from build123d import *

# Parameters (mm, degrees)
BOSS_EXTRUDE1_DEPTH = 1.5


with BuildPart() as part:
    # Sketch1 → Revolve1 (revolve)
    with BuildSketch(Plane.XY, mode=Mode.PRIVATE) as revolve1_sk:
        with BuildLine():
            Line((0, 0), (1.775, 0))
            Line((1.775, 0), (1.775, 6.5))
            Line((1.775, 6.5), (2.775, 6.5))
            ThreePointArc((2.775, 6.5), (2.302554278, 6.609277193), (1.818611947, 6.640038943))
            Line((1.818611947, 6.640038943), (0, 6.640038943))
            Line((0, 6.640038943), (0, 0))
        make_face()
    revolve(revolve1_sk.sketch.rotate(Axis((0, 0, 0), (0, 1, 0)), 90), axis=Axis((0, 0, 0), (0, 1, 0)))

    # Sketch2 → Boss-Extrude1 (add)
    with BuildSketch(Plane(origin=(0, 6.640038943, 0), x_dir=(1, 0, 0), z_dir=(0, 1, 0))):
        Polygon((1.349267315, 1.604637118), (-0.71502285, 1.97081833), (-2.064290165, 0.366181213), (-1.349267315, -1.604637118), (0.71502285, -1.97081833), (2.064290165, -0.366181213), align=None)
    extrude(amount=BOSS_EXTRUDE1_DEPTH)

    # Sketch3 → Cut-Revolve1 (revolve, cut)
    with BuildSketch(Plane.XY, mode=Mode.PRIVATE) as cut_revolve1_sk:
        Polygon((1.11158303, 8.796006759), (2.422382115, 7.573543033), (2.422382115, 8.796006759), align=None)
    revolve(cut_revolve1_sk.sketch.rotate(Axis((0, 0, 0), (0, 1, 0)), 90), axis=Axis((0, 0, 0), (0, 1, 0)), mode=Mode.SUBTRACT)


solid = part.part
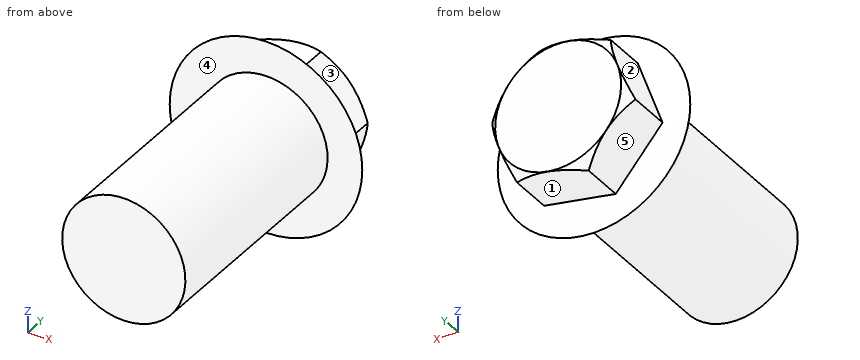
Geometry check sheet. Reference: the model listing, model coordinates, mm. Face numbers are marked on the shaded views. A direction names the side the tool comes from. Round coordinates to 2 decimals unless told otherwise and drop trailing zeros. Order: outer loops, then holes, each group sorted by start corner. A loop starts at its lowest first (then second) coordinate and runs counter-clockwise, first axis right, second up. Notation, with made-up numbers: M 73,85 L 124,85 A15 cw 124,112 Z; hole C 81.5,26.25 d4. An arc over 180 degrees is marked long. Write each question's results on one line, items separated by ' | '. Start each with the question number.
1. Material ranges on L1, parallel to Z at x = -0.6, y = 3.75; L2, parallel to X at y = 3.5, z = 0 (3 decimals); L3, parallel to X at y = 5.5, z = -0.35, recorded low to high. Write a range as from..to.
2. Set-up check for the marked faces 1, 2, 3, 4 and 5: record each of +Z, -Z, +X, -X, +Y, -Y from which the full face is reachable in a straight line by a thin tool's end or side.
3. Cross-section at A-A on y = 1.25. Record the boundary of the cut face in (x, z) (3 decimals), plus the area to 3 significant figures.
Resolved:
1) L1: -1.67..1.67 | L2: -1.775..1.775 | L3: -1.74..1.74
2) face 1: -Z, +X, +Y | face 2: +Z, -X, +Y | face 3: +Z, +X, +Y | face 4: -Y | face 5: -Z, -X, +Y
3) outline: C 0,0 d3.55 | area: 9.90 mm2
